from build123d import *

# Parameters (mm, degrees)
F1_DEPTH = 30
F2_R     = 2.25
F3_DEPTH = 7


with BuildPart() as f1:
    # F0 (on Front) → F1 (new body)
    with BuildSketch(Plane.XZ):
        with BuildLine():
            Line((-12, -13.1), (-12, 13.1))
            Line((-12, 13.1), (-8.5, 16.6))
            Line((-8.5, 16.6), (-8.5, 20.1))
            Line((-8.5, 20.1), (-12, 23.6))
            Line((-12, 23.6), (-19, 23.6))
            Line((-19, 23.6), (-19, -27.1))
            Line((-19, -27.1), (0, -27.1))
            Line((0, -27.1), (19, -27.1))
            Line((19, -27.1), (81, -27.1))
            Line((81, -27.1), (100, -27.1))
            Line((100, -27.1), (119, -27.1))
            Line((119, -27.1), (119, 23.6))
            Line((119, 23.6), (112, 23.6))
            Line((112, 23.6), (108.5, 20.1))
            Line((108.5, 20.1), (108.5, 16.6))
            Line((108.5, 16.6), (112, 13.1))
            Line((112, 13.1), (112, -13.1))
            Line((112, -13.1), (105, -20.1))
            Line((105, -20.1), (95, -20.1))
            Line((95, -20.1), (88, -13.1))
            Line((88, -13.1), (88, 13.1))
            Line((88, 13.1), (91.5, 16.6))
            Line((91.5, 16.6), (91.5, 20.1))
            Line((91.5, 20.1), (88, 23.6))
            Line((88, 23.6), (81, 23.6))
            Line((81, 23.6), (81, -15.1))
            ThreePointArc((81, -15.1), (79.535534, -18.635534), (76, -20.1))
            Line((76, -20.1), (24, -20.1))
            ThreePointArc((24, -20.1), (20.464466, -18.635534), (19, -15.1))
            Line((19, -15.1), (19, 23.6))
            Line((19, 23.6), (12, 23.6))
            Line((12, 23.6), (8.5, 20.1))
            Line((8.5, 20.1), (8.5, 16.6))
            Line((8.5, 16.6), (12, 13.1))
            Line((12, 13.1), (12, -13.1))
            Line((12, -13.1), (5, -20.1))
            Line((5, -20.1), (-5, -20.1))
            Line((-5, -20.1), (-12, -13.1))
        make_face()
    extrude(amount=F1_DEPTH)

    # F2 (on face) → F3 (cut, through all)
    with BuildSketch(Plane.XY.offset(-20.1)):
        with Locations((34, -15)):
            Circle(F2_R)
        with Locations((66, -15)):
            Circle(F2_R)
    extrude(amount=-F3_DEPTH, mode=Mode.SUBTRACT)


solid = f1.part
Build history of the part. All positions in model axes, mm. A direction names the side the tool comes from. Coordinates: 2 decimals unless noted, no trailing zeros. Order: outer loops, then holes, each group sorted by start corner. A loop starts at its lowest first (then second) coordinate and runs counter-clockwise, first axis right, second up. Notation, with made-up numbers: (39, -2.5) - (98, -2.5) arc R21 cw to (98, 14.5) - close; hole circle Ø6 at (74, 54.5). An arc over 180 degrees is marked (long way). Write each question's results on one line, items separated by ' | '. Start each with the question number.
Item 1: Flat gauge pins, fed straight in: pin 1 (11 mm diameter, centred on x = 102.5, y = -21, fed in from +Z); pin 2 (15 mm diameter, centred on x = 62.5, y = -9.5, fed in from +Z). Where does each tip first touch, or does it go through?
Item 2: Band-saw the part on D-D on y = -15. State how many separate pieces and enclosed holes the cut face has, and give its area (3 significant figures).
Item 3: Wall check: probe 1 along X at (y, z) = (-5.5, 18); probe 2 along X at (y, z) = (-20, -5); probe 3 along Y at (x, z) = (66, -23). Give the ranges that are in metal, low to high. Write a range as [from, to].
Item 4: Tool access for faces 4 (the face through (79.57, -14.79, -18.6)), 5 (the face through (8.5, -14.8, -16.6)), 6 (the face through (16, -15, 23.6)): list every direction of +Z, -Z, +X, -X, +Y, -Y with a clear straight run to the whole face (end or side of a thin tool).
Item 5: Band-saw the part on A-A on z = 11. Write the cut outline in (x, y), and give its area (3 significant figures).
Item 6: Mould opens along X. For faces 1 (the face through (119, -15, -2)), 2 (the face through (12, -15, 0)), 3 (the face through (116, -15, 23.6)) say: released by +X, released by -X, zero draft, split by the parting line, or undercut.
Item 7: Band-saw the part on B-B on x = 34. Write the cut outline in (y, z), and give its area (4 significant figures).
Numbers:
1) pin 1: z = -17.1 | pin 2: z = -20.1
2) separate pieces: 3 | enclosed holes: 0 | area: 2,330 mm^2
3) probe 1: [-19, -8.5], [8.5, 19], [81, 91.5], [108.5, 119] | probe 2: [-19, -12], [12, 19], [81, 88], [112, 119] | probe 3: [-30, -17.25], [-12.75, 0]
4) face 4: +Z, +Y, -Y | face 5: +Y, -Y | face 6: +Z, +X, -X, +Y, -Y
5) outline: (-19, -30) - (-12, -30) - (-12, 0) - (-19, 0) - close; (12, -30) - (19, -30) - (19, 0) - (12, 0) - close; (81, -30) - (88, -30) - (88, 0) - (81, 0) - close; (112, -30) - (119, -30) - (119, 0) - (112, 0) - close | area: 840 mm^2
6) face 1: released by +X | face 2: undercut | face 3: zero draft
7) outline: (-30, -27.1) - (-17.25, -27.1) - (-17.25, -20.1) - (-30, -20.1) - close; (-12.75, -27.1) - (0, -27.1) - (0, -20.1) - (-12.75, -20.1) - close | area: 178.5 mm^2
